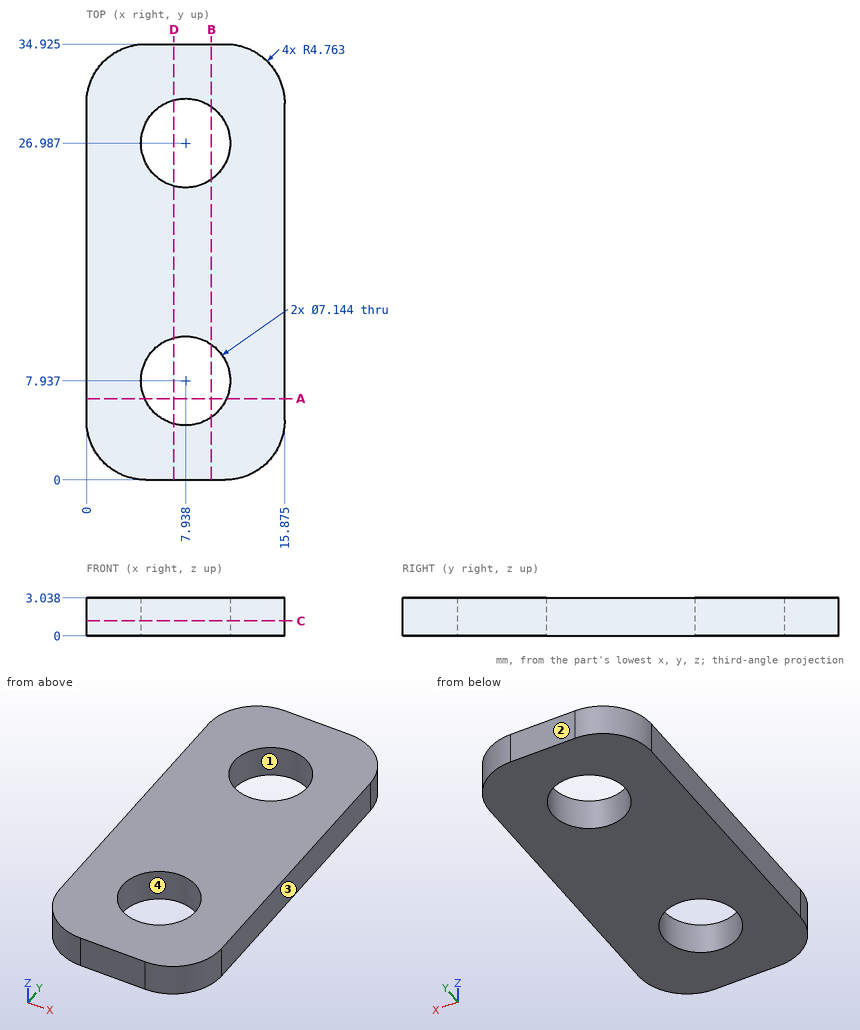
Study the drawing (mm; zero at the part's minimum x, y, z) and answer. Coordinates: 2 decimals unless noted, no trailing zeros. Order: outer loops, then holes, each group sorted by start corner. A loop starts at its lowest first (then second) coordinate and runs counter-clockwise, first axis right, second up. Notation, with made-up numbers: (7.5, -6) -> (31.5, -6) arc R38 cw to (31.5, 32) -> close; hole circle Ø4 at (23, -12). An arc over 180 degrees is marked (long way). Answer in a Markdown table with one row per item. Add a question column.
Item 1: Find section A-A (y = 6.5). Write down the section's boundary in (x, z) (1 decimal).
Item 2: Determine the mould class of the marked faces 1, 2, 3 and 4 for opening direction Y: +Y half, -Y half, draft (parallel to the pull), parting line (faces both ways), or undercut.
Item 3: This flat-tipped pin is pushed along its axis until it touches: P1, Ø2, axis at x = 6.5, y = 8, coming from the +Z side (3 decimals). Where does it stop, or does it pass through?
Item 4: Find section B-B (x = 10). Write down the section's boundary in (y, z) (1 decimal).
Item 5: Find section D-D (x = 7). Write down the section's boundary in (y, z) (1 decimal).
Item 6: Find section C-C (z = 1.2). Write down the section's boundary in (x, y) (1 decimal).
Item 7: Find the intervals of material crossed by L1, parallel to Y at x = 10.25, z = 2.35 (1 decimal); L2, parallel to Y at x = 9.25, z = 2.2 (1 decimal); L3, parallel to X at y = 26.5, z = 1.4 (1 decimal), in increasing order. Write a range as from..to.
Result set:
| question | item | result |
|---|---|---|
| 1 | outline | (0, 0) -> (4.7, 0) -> (4.7, 3) -> (0, 3) -> close; (11.2, 0) -> (15.9, 0) -> (15.9, 3) -> (11.2, 3) -> close |
| 2 | face 1 | undercut |
| 2 | face 2 | +Y half |
| 2 | face 3 | draft |
| 2 | face 4 | undercut |
| 3 | P1 | passes through |
| 4 | outline | (0, 0) -> (5, 0) -> (5, 3) -> (0, 3) -> close; (10.9, 0) -> (24.1, 0) -> (24.1, 3) -> (10.9, 3) -> close; (29.9, 0) -> (34.9, 0) -> (34.9, 3) -> (29.9, 3) -> close |
| 5 | outline | (0, 0) -> (4.5, 0) -> (4.5, 3) -> (0, 3) -> close; (11.4, 0) -> (23.5, 0) -> (23.5, 3) -> (11.4, 3) -> close; (30.4, 0) -> (34.9, 0) -> (34.9, 3) -> (30.4, 3) -> close |
| 6 | outline | (0, 4.8) arc R4.8 ccw to (4.8, 0) -> (11.1, 0) arc R4.8 ccw to (15.9, 4.8) -> (15.9, 30.2) arc R4.8 ccw to (11.1, 34.9) -> (4.8, 34.9) arc R4.8 ccw to (0, 30.2) -> close; hole circle Ø7.1 at (7.9, 7.9); hole circle Ø7.1 at (7.9, 27) |
| 7 | L1 | y = 0..5.2, 10.7..24.3, 29.7..34.9 |
| 7 | L2 | y = 0..4.6, 11.3..23.7, 30.3..34.9 |
| 7 | L3 | x = 0..4.4, 11.5..15.9 |
